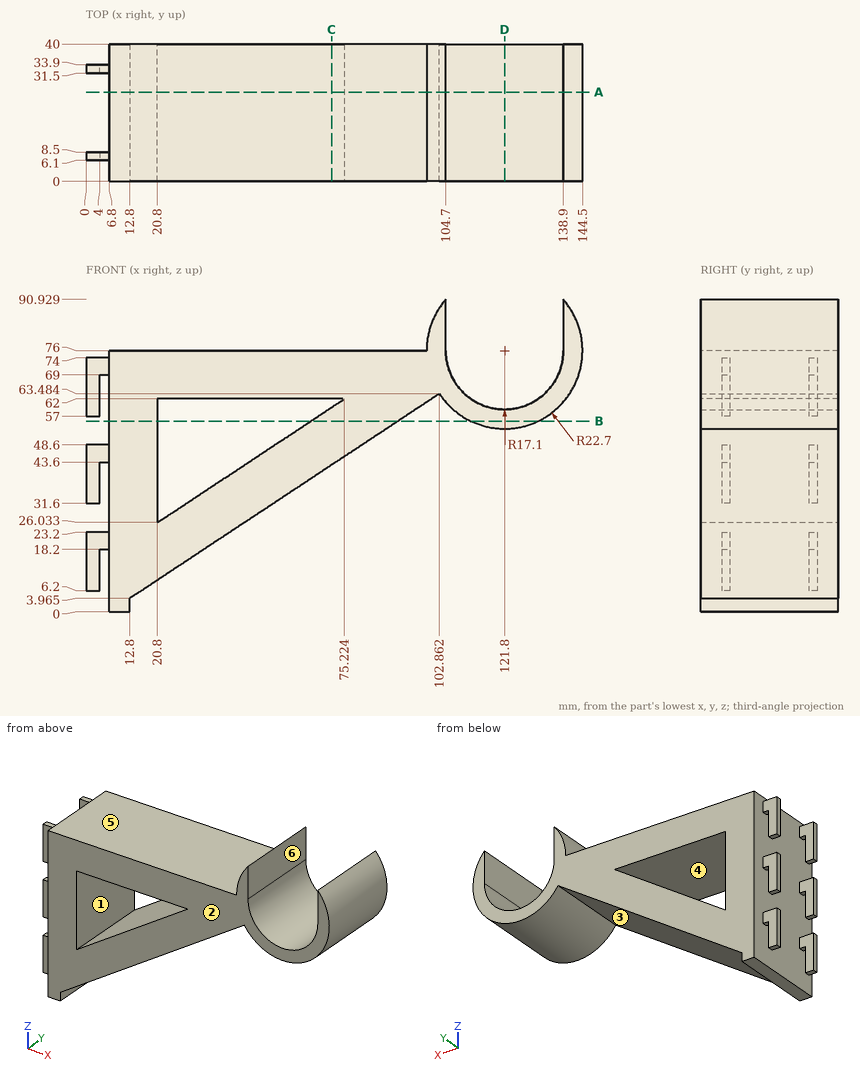
The figure shows three views and two pictorial views of one solid part (mm, origin at its lowest corner). Answer the questions. A direction names the side the tool comes from. Give positions to 0.01 mm unless a question says otherwise; leave off trailing zeros. Write each loop counter-clockwise with the first axis right and the second up, starting at its lowest first coordinate (ties: lowest second). Pieces come first, ordered by that corner, then holes. Notation, with made-up numbers: (9, 81) -> (17, 81) arc R26 ccw to (17, 104) -> close; hole circle Ø4 at (62, 44). An arc over 180 degrees is marked (long way). Answer as a JSON object with one key per item and string values.
1) Section B-B on z = 55.5 is taken. Write down the section's boundary in (x, y).
Findings below:
{"outline": "(6.8, 0) -> (20.8, 0) -> (20.8, 40) -> (6.8, 40) -> close; (65.39, 0) -> (90.78, 0) -> (90.78, 40) -> (65.39, 40) -> close; (112.05, 0) -> (131.55, 0) -> (131.55, 40) -> (112.05, 40) -> close"}
2) Section D-D on x = 121.8 is taken. Write down the section's boundary in (y, z).
Findings below:
{"outline": "(0, 53.3) -> (40, 53.3) -> (40, 58.9) -> (0, 58.9) -> close"}
3) For a pull along X with two mould halves and no side action, classify the marked faces 1 and 2 as pulls with the +X half, pulls with the -X half, needs draft (parallel to the pull), parting line crosses it, or undercut.
Findings below:
{"face 1": "undercut", "face 2": "needs draft"}
4) Section A-A on y = 26 is taken. Write down the section's boundary in (x, z) (1 decimal), then the cut area to 3 significant figures.
Findings below:
{"outline": "(6.8, 0) -> (12.8, 0) -> (12.8, 4) -> (102.9, 63.5) arc R22.7 ccw (long way) to (138.9, 90.9) -> (138.9, 76) arc R17.1 cw to (104.7, 76) -> (104.7, 90.9) arc R22.7 ccw to (99.1, 76) -> (6.8, 76) -> close; hole (20.8, 26) -> (75.2, 62) -> (20.8, 62) -> close", "area": "3,720 mm^2"}
5) A tool of negligible diameter and unlimited length cuts with its end or side. For the marked faces 3, 4, 5 and 6, from which of +Z, -Z, +X, -X, +Y, -Y can it reach the whole face along a straight path? Write none if from no direction.
Findings below:
{"face 3": "-Z, +Y, -Y", "face 4": "+Y, -Y", "face 5": "+Z, -X, +Y, -Y", "face 6": "+Z, +Y, -Y"}
6) Flat-ended cylindrical pins translate along their axes: pin 1 Ø6 at (x, y) = (16.5, 35) entering from +Z; pin 2 Ø2.5 at (x, y) = (5, 32.5) entering from -Z; pin 3 Ø3.5 at (x, z) = (3.5, 13.5) entering from -Y. Find the tip coordinate at first contact, or state that the pin passes through.
Findings below:
{"pin 1": "stops at z = 76", "pin 2": "stops at z = 6.2", "pin 3": "stops at y = 6.1"}
7) Straight lines are drawn through the part: probe 1 along X at (y, z) = (33, 52) (1 decimal); probe 2 along Z at (x, y) = (62.5, 10); probe 3 along X at (y, z) = (19, 27) (1 decimal). For each, find the intervals that lie inside material, in ascending order. Write a range as from..to.
Findings below:
{"probe 1": "x = 6.8..20.8, 60.1..85.5", "probe 2": "z = 36.81..53.59, 62..76", "probe 3": "x = 6.8..20.8, 22.3..47.7"}
8) Section C-C on x = 71.5 is taken. Write down the section's boundary in (y, z), then the cut area to 3 significant figures.
Findings below:
{"outline": "(0, 42.76) -> (40, 42.76) -> (40, 59.54) -> (0, 59.54) -> close; (0, 62) -> (40, 62) -> (40, 76) -> (0, 76) -> close", "area": "1,230 mm^2"}
